```python
from build123d import *

# Parameters (mm, degrees)
SKETCH1_R           = 2.25
BOSS_EXTRUDE1_DEPTH = 2
FILLET1_R           = 10.25
FILLET2_R           = 2
SKETCH2_R           = 1.5
SKETCH2_W           = 4
SKETCH2_H           = 2
CUT_EXTRUDE1_DEPTH  = 2
FILLET3_R           = 8


with BuildPart() as part:
    # Sketch1 → Boss-Extrude1 (new body)
    with BuildSketch(Plane(origin=(0, 0, 0), x_dir=(1, 0, 0), z_dir=(0, 1, 0))):
        Polygon((0, 0), (32.5, 0), (32.5, -10.25), (60.5, -10.25), (60.5, -0.75), (60.5, 21.25), (60.5, 30.75), (32.5, 30.75), (32.5, 20.5), (0, 20.5), align=None)
        with Locations(Location((10.25, 10.25, 0), (0, 0, 270))):
            Circle(SKETCH1_R, mode=Mode.SUBTRACT)
    extrude(amount=BOSS_EXTRUDE1_DEPTH)

    # Fillet1
    fillet1_edges = [part.edges().sort_by_distance(p)[0] for p in [
        (0, 1, -20.5),
        (0, 1, 0),
    ]]
    fillet(fillet1_edges, radius=FILLET1_R - 0.0001)  # a hair under: the kernel refuses the full size

    # Fillet2
    fillet2_edges = [part.edges().sort_by_distance(p)[0] for p in [
        (32.5, 1, -30.75),
        (60.5, 1, -30.75),
        (60.5, 1, 10.25),
        (32.5, 1, 10.25),
    ]]
    fillet(fillet2_edges, radius=FILLET2_R)

    # Sketch2 → Cut-Extrude1 (cut)
    with BuildSketch(Plane(origin=(0, 2, 0), x_dir=(1, 0, 0), z_dir=(0, 1, 0))):
        with Locations(Location((46.5, 28.75, 0), (0, 0, 270))):
            Circle(SKETCH2_R)
        with Locations(Location((46.5, 10.25, 0), (0, 0, 270))):
            Circle(SKETCH2_R)
        with Locations(Location((46.5, -8.25, 0), (0, 0, 270))):
            Circle(SKETCH2_R)
        with Locations((39.5, 28.75)):
            Rectangle(SKETCH2_W, SKETCH2_H)
        with Locations((53.5, 28.75)):
            Rectangle(SKETCH2_W, SKETCH2_H)
        with Locations((39.5, 10.25)):
            Rectangle(SKETCH2_W, SKETCH2_H)
        with Locations((53.5, 10.25)):
            Rectangle(SKETCH2_W, SKETCH2_H)
        with Locations((39.5, -8.25)):
            Rectangle(SKETCH2_W, SKETCH2_H)
        with Locations((53.5, -8.25)):
            Rectangle(SKETCH2_W, SKETCH2_H)
    extrude(amount=-CUT_EXTRUDE1_DEPTH, mode=Mode.SUBTRACT)

    # Fillet3
    fillet3_edges = [part.edges().sort_by_distance(p)[0] for p in [
        (32.5, 1, -20.5),
        (32.5, 1, 0),
    ]]
    fillet(fillet3_edges, radius=FILLET3_R)


solid = part.part
```
Build history of the part. All positions in model axes, mm. A direction names the side the tool comes from. Give positions to 0.01 mm unless a question says otherwise; leave off trailing zeros. Loops run counter-clockwise (first coordinate to the right, second up) from the corner with the lowest first, then second, coordinate; pieces in that order, holes last.
Item 1: Which spindle directions (+Z, -Z, +X, -X, +Y, -Y) get a long thin tool onto all of the face, cutting with end or side? Do faces 5 (the face through (17, 1, -20.5)), 6 (the face through (41.5, 1, 8)), 7 (the face through (37, 2, -11)). Say none if no direction does.
Answers follow:
face 5: -Z, -X, +Y, -Y
face 6: +Y, -Y
face 7: +Z, -Z, +X, -X, +Y
Item 2: Flat gauge pin, fed straight in: pin 1 (1 mm diameter, centred on y = 1, z = -29, fed in from -X). Where does the tip first touch, or does it go through?
Answers follow:
pin 1: stops at x = 32.5
Item 3: Slice it at D-D, the plane z = -6. List the corners of the cut face in (x, y).
Answers follow:
outline: (0.92, 0) - (60.5, 0) - (60.5, 2) - (0.92, 2) - close
Item 4: Drill centre lines: line 1 (X direction, y = 1, z = -10.25); line 2 (Z direction, x = 53.5, y = 1.1); line 3 (X direction, y = 0.8, z = 8.25). Where is each one in solid material? Low to high.
Answers follow:
line 1: x = 0 to 8, 12.5 to 37.5, 41.5 to 45, 48 to 51.5, 55.5 to 60.5
line 2: z = -30.75 to -29.75, -27.75 to -11.25, -9.25 to 7.25, 9.25 to 10.25
line 3: x = 32.5 to 37.5, 41.5 to 45, 48 to 51.5, 55.5 to 60.5
Item 5: Slice it at A-A, the plane x = 38.5. List the corners of the cut face in (y, z), and give its area (3 significant figures).
Answers follow:
outline: (0, -30.75) - (2, -30.75) - (2, -29.75) - (0, -29.75) - close; (0, -27.75) - (2, -27.75) - (2, -11.25) - (0, -11.25) - close; (0, -9.25) - (2, -9.25) - (2, 7.25) - (0, 7.25) - close; (0, 9.25) - (2, 9.25) - (2, 10.25) - (0, 10.25) - close
area: 70.0 mm2
Item 6: Slice it at B-B, the plane y = 1.55. Give the number of separate pieces and of enclosed holes in the cut face, and give its area (3 significant figures).
Answers follow:
separate pieces: 1
enclosed holes: 10
area: 1,710 mm2
Item 7: Pull direction Z, two halves, no side cores. Call faces 1 (the face through (59.93, 1.01, -30.15)), 2 (the face through (55.5, 1, -29)), 3 (the face through (33.07, 1.01, 9.65)), 4 (the face through (41.5, 1, -29)): released by +Z, released by -Z, zero draft, split by the parting line, or undercut.
Answers follow:
face 1: released by -Z
face 2: undercut
face 3: released by +Z
face 4: undercut
Item 8: Slice it at C-C, the plane x = 46.5. List the corners of the cut face in (y, z), and give its area (3 significant figures).
Answers follow:
outline: (0, -30.75) - (2, -30.75) - (2, -30.25) - (0, -30.25) - close; (0, -27.25) - (2, -27.25) - (2, -11.75) - (0, -11.75) - close; (0, -8.75) - (2, -8.75) - (2, 6.75) - (0, 6.75) - close; (0, 9.75) - (2, 9.75) - (2, 10.25) - (0, 10.25) - close
area: 64.0 mm2
